The model under review builds one solid part; all positions refer to its coordinate system, in mm. A direction names the side the tool comes from. Round coordinates to 2 decimals unless told otherwise and drop trailing zeros. Loops run counter-clockwise (first coordinate to the right, second up) from the corner with the lowest first, then second, coordinate; pieces in that order, holes last. Notation, with made-up numbers: M 43,78 L 56,78 A20 cw 56,85 Z; hole C 7,63.5 d2. An arc over 180 degrees is marked long. Return JSON: item names as keys, results as strings. Group by question number.
Q1. Consider section A-A (y = 51). State the section outline as (x, z) points, and give its area (3 significant figures).
Q2. To check wall thickness, follow line 1 along Y through (x, z) = (9, 23.5); line 2 along Z through (x, y) = (16.5, 50.5); line 3 along Y through (x, z) = (16.3, 13.5). State the ranges of each line that lie inside material, in increasing order.
Q3. Consider section C-C (y = 30.5). State the section outline as (x, z) points.
Q4. Clearance check with flat-ended pins moving along their axes: pin 1 Ø6 at (x, z) = (15.5, 13) entering from +Y; pin 2 Ø5.5 at (x, z) = (9, 13.5) entering from -Y. State where each tip first meets the part, or that it passes through.
Q5. Consider section D-D (z = 13.5). State the section outline as (x, y) points, and give its area (3 significant figures).
Q6. Draft analysis for pull direction Z (two halves, no side actions). For faces 5 (the face through (0, 31, 13)), 6 (the face through (9, 31, 0)), 7 (the face through (6.9, 12.4, 8)), state which applies: pulls with the +Z half, pulls with the -Z half, needs draft (parallel to the pull), parting line crosses it, or undercut.
Q7. Consider section B-B (x = 14.75). State the section outline as (y, z) points.
Q8. For faces 1 (the face through (9, 41, 14)), 2 (the face through (9, 20, 14)), 3 (the face through (13, 31, 14)), 4 (the face through (9, 54, 4)), list the 3-axis set-ups (+Z, -Z, +X, -X, +Y, -Y) from which the entire face can be reached by the end or side of a thin tool; tool diameter is ignored.
Autodesk Inventor part; units mm, degrees
ref_plane "YZ Plane" through (0, 0, 0) normal (1, 0, 0) x (0, 1, 0)
ref_plane "XZ Plane" through (0, 0, 0) normal (0, 1, 0) x (-1, 0, 0)
ref_plane "XY Plane" through (0, 0, 0) normal (0, 0, 1) x (1, 0, 0)
sketch "Sketch1" plane through (0, 0, 0) normal (0, 0, 1) x (1, 0, 0)
  line L0 (0, 0) -> (18, 0)
  line L1 (18, 0) -> (18, 61)
  line L2 (18, 61) -> (0, 61)
  line L3 (0, 61) -> (0, 0)
  dimension "d0" = 18
  dimension "d1" = 61
extrude "Extrusion1" add sketch "Sketch1" along normal blind 27
sketch "Sketch2" plane through (0, 0, 0) normal (-1, 0, 0) x (0, 0, 1)
  line L0 (0, 61) -> (27, 61)
  line L1 (8, 61) -> (19, 61)
  line L2 (19, 61) -> (19, 41)
  line L3 (19, 41) -> (8, 41)
  line L4 (8, 41) -> (8, 61)
  line L5 (-7.2771, 30.5) -> (-16.8885, 30.5) construction
  line L6 (0, 61) -> (0, 0) construction
  line L7 (8, 0) -> (19, 0)
  line L8 (19, 0) -> (19, 20)
  line L9 (19, 20) -> (8, 20)
  line L10 (8, 20) -> (8, 0)
  point P0 (-12.0828, 30.5)
  point P1 (0, 30.5)
  point P2 (13.5, 61)
  point P3 (13.5, 61)
  dimension "d4" = 11
  dimension "d5" = 20
extrude "Extrusion2" cut sketch "Sketch2" against normal through all
sketch "Sketch3" plane through (0, 0, 27) normal (0, 0, 1) x (1, 0, 0)
  circle A0 centre (9, 51) radius 3
  line L0 (-26.5753, 30.5) -> (-43.832, 30.5) construction
  line L1 (0, 61) -> (0, 0) construction
  circle A1 centre (9, 10) radius 3
  line L2 (18, 61) -> (0, 61) construction
  line L3 (0, 41) -> (18, 41) construction
  line L4 (18, 61) -> (0, 61) construction
  line L5 (0, 61) -> (0, 41) construction
  line L6 (0, 41) -> (18, 41) construction
  line L7 (18, 41) -> (18, 61) construction
  point P0 (-35.2037, 30.5)
  point P1 (0, 30.5)
  point P2 (0, 51)
  point P3 (9, 61)
  dimension "d8" = 6
extrude "Extrusion3" cut sketch "Sketch3" against normal through all
sketch "Sketch4" plane through (18, 0, 0) normal (1, 0, 0) x (0, 0, -1)
  circle A0 centre (-13.5, 30.5) radius 6.5
  line L0 (-27, 0) -> (-27, 61)
  line L1 (-8, 41) -> (-19, 41)
  point P0 (0, 0)
  point P1 (-27, 30.5)
  point P2 (-13.5, 41)
  dimension "bearingdiameter" = 13
extrude "Extrusion4" cut sketch "Sketch4" against normal blind 5
properties part number "hinge"
Values:
{
 "1": {"outline": "M 0,0 L 6,0 L 6,8 L 0,8 Z; M 0,19 L 6,19 L 6,27 L 0,27 Z; M 12,0 L 18,0 L 18,8 L 12,8 Z; M 12,19 L 18,19 L 18,27 L 12,27 Z", "area": "192 mm2"},
 "2": {"line 1": "y = 0 to 7, 13 to 48, 54 to 61", "line 2": "z = 0 to 8, 19 to 27", "line 3": "y = 20 to 24, 37 to 41"},
 "3": {"outline": "M 0,0 L 18,0 L 18,7 L 13,7 L 13,20 L 18,20 L 18,27 L 0,27 Z"},
 "4": {"pin 1": "stops at y = 41", "pin 2": "stops at y = 20"},
 "5": {"outline": "M 0,20 L 18,20 L 18,24 L 13,24 L 13,37 L 18,37 L 18,41 L 0,41 Z", "area": "313 mm2"},
 "6": {"face 5": "needs draft", "face 6": "pulls with the -Z half", "face 7": "undercut"},
 "7": {"outline": "M 0,0 L 61,0 L 61,8 L 41,8 L 41,19 L 61,19 L 61,27 L 0,27 L 0,19 L 20,19 L 20,8 L 0,8 Z; hole C 30.5,13.5 d13"},
 "8": {"face 1": "+X, -X, +Y", "face 2": "+X, -X, -Y", "face 3": "+X", "face 4": "+Z, -Z"}
}
